The model under review builds one solid part; all positions refer to its coordinate system, in mm. Coordinates: 2 decimals unless noted, no trailing zeros. Loops run counter-clockwise (first coordinate to the right, second up) from the corner with the lowest first, then second, coordinate; pieces in that order, holes last. Notation, with made-up numbers: (-12, -12) - (42, -12) arc R19 cw to (42, 7) - close; hole circle Ø10 at (-40, 89). An arc over 180 degrees is marked (long way). Use a Markdown table: item, result. Add a question column.
1) To check wall thickness, follow L1, parallel to Y at x = 0, z = 1.5 (3 decimals); L2, parallel to X at y = 1, z = 5.5; L3, parallel to Y at x = 5.5, z = 1.75. State the ranges of each line that lie inside material, in increasing order. Write a range as [from, to].
2) Add section C-C, the plane z = 5. Give the boundary of the cut face in (x, y) (3 decimals), and give its area (3 significant figures).
3) The part is to be moulded in two halves that separate along Y. For faces 1 (the cylindrical face through (-1.38, -6.2, 2.74)), 2 (the cylindrical face through (-0.69, -3.1, 3.53)), 3 (the flat face through (2, -3, 7.144)), say which applies: pulls with the +Y half, pulls with the -Y half, needs draft (parallel to the pull), parting line crosses it, or undercut.
4) Clearance check with a flat-ended pin moving along its axis: pin 1 (4 mm diameter, centred on x = 3, z = 1.5, fed in from +Y). State where the tip first meets the part, or that it passes through.
```python
from build123d import *

# Parameters (mm, degrees)
F0_R     = 6.35
F0_R_2   = 3.175
F1_DEPTH = 7.14375
F2_SIZE  = 1.5875
F3_SIZE  = 0.254


with BuildPart() as f1:
    # F0 (on Top) → F1 (new body)
    with BuildSketch(Plane.XY):
        Circle(F0_R)
        Circle(F0_R_2, mode=Mode.SUBTRACT)
    extrude(amount=F1_DEPTH)

    # F2
    f2_edges = [f1.edges().sort_by_distance(p)[0] for p in [
        (-6.35, 0, 7.14375),
    ]]
    chamfer(f2_edges, length=F2_SIZE)

    # F3
    f3_edges = [f1.edges().sort_by_distance(p)[0] for p in [
        (-3.175, 0, 7.14375),
        (-3.175, 0, 0),
    ]]
    chamfer(f3_edges, length=F3_SIZE)


solid = f1.part
```
From the geometry:
| question | item | result |
|---|---|---|
| 1 | L1 | y = [-6.35, -3.175], [3.175, 6.35] |
| 1 | L2 | x = [-6.27, -3.01], [3.01, 6.27] |
| 1 | L3 | y = [-3.17, 3.17] |
| 2 | outline | circle Ø12.7 at (0, 0); hole circle Ø6.35 at (0, 0) |
| 2 | area | 95.0 mm^2 |
| 3 | face 1 | parting line crosses it |
| 3 | face 2 | undercut |
| 3 | face 3 | needs draft |
| 4 | pin 1 | stops at y = 6.27 |
